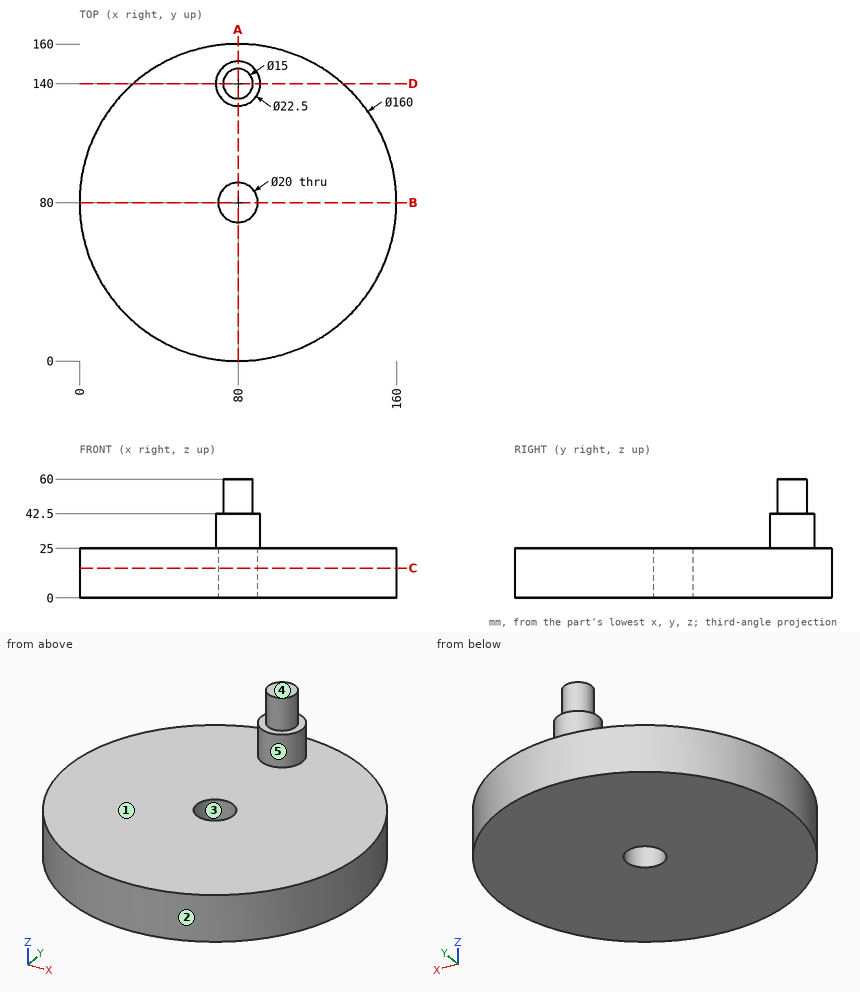
Input: dimensioned drawing with shaded views. Units: mm. Origin: part minimum x, y, z. A direction names the side the tool comes from. Give positions to 0.01 mm unless a question says otherwise; leave off trailing zeros. Loops run counter-clockwise (first coordinate to the right, second up) from the corner with the lowest first, then second, coordinate; pieces in that order, holes last. Notation, with made-up numbers: (8.5, 35) -> (33.5, 35) arc R5 cw to (33.5, 41) -> close; hole circle Ø9 at (-15.5, -2.75). An arc over 180 degrees is marked (long way). Use a Markdown table: item, result. Add a question column.
1) Section query A-A, the plane x = 80. Return the cut outline in (y, z), then the cut area to 3 significant figures.
2) Section query D-D, the plane y = 140. Return the cut outline in (x, z).
3) Pull-direction query (Y, two-part tool) for the marked faces 1, 2 and 3; classes: +Y half, -Y half, draft (parallel to the pull), parting line (faces both ways), or undercut.
4) Reachability of the marked faces 4 and 5 from +Z, -Z, +X, -X, +Y, -Y: full face, straight path, thin tool, end or side. Return the list, or none.
5) Section query B-B, the plane y = 80. Return the cut outline in (x, z), then the cut area to 3 significant figures.
6) Line query: line 1 along Y through (x, z) = (80, 9); line 2 along Z through (x, y) = (108.5, 88); line 3 along X through (y, z) = (8, 15.5). Output: solid intervals per line, ascending. Write a range as [from, to].
7) First-contact query: pin 1 (12 mm diameter, centred on x = 66, y = 54, fed in from +Z); pin 2 (8 mm diameter, centred on y = 123, z = 12, fed in from +X); pin 3 (12 mm diameter, centred on x = 36, z = 6.5, fed in from -Y); pin 4 (18 mm diameter, centred on x = 80, y = 80, fed in from +Z). Flat tips, straight axial feed; report the tip coordinate or a pass-through.
8) Section query C-C, the plane z = 15. Return the cut outline in (x, y).
Numbers:
| question | item | result |
|---|---|---|
| 1 | outline | (0, 0) -> (70, 0) -> (70, 25) -> (0, 25) -> close; (90, 0) -> (160, 0) -> (160, 25) -> (151.25, 25) -> (151.25, 42.5) -> (147.5, 42.5) -> (147.5, 60) -> (132.5, 60) -> (132.5, 42.5) -> (128.75, 42.5) -> (128.75, 25) -> (90, 25) -> close |
| 1 | area | 4,160 mm2 |
| 2 | outline | (27.08, 0) -> (132.92, 0) -> (132.92, 25) -> (91.25, 25) -> (91.25, 42.5) -> (87.5, 42.5) -> (87.5, 60) -> (72.5, 60) -> (72.5, 42.5) -> (68.75, 42.5) -> (68.75, 25) -> (27.08, 25) -> close |
| 3 | face 1 | draft |
| 3 | face 2 | parting line |
| 3 | face 3 | undercut |
| 4 | face 4 | +Z, +X, -X, +Y, -Y |
| 4 | face 5 | +Z |
| 5 | outline | (0, 0) -> (70, 0) -> (70, 25) -> (0, 25) -> close; (90, 0) -> (160, 0) -> (160, 25) -> (90, 25) -> close |
| 5 | area | 3,500 mm2 |
| 6 | line 1 | y = [0, 70], [90, 160] |
| 6 | line 2 | z = [0, 25] |
| 6 | line 3 | x = [45.13, 114.87] |
| 7 | pin 1 | stops at z = 25 |
| 7 | pin 2 | stops at x = 149.85 |
| 7 | pin 3 | stops at y = 9.6 |
| 7 | pin 4 | passes through |
| 8 | outline | circle Ø160 at (80, 80); hole circle Ø20 at (80, 80) |
